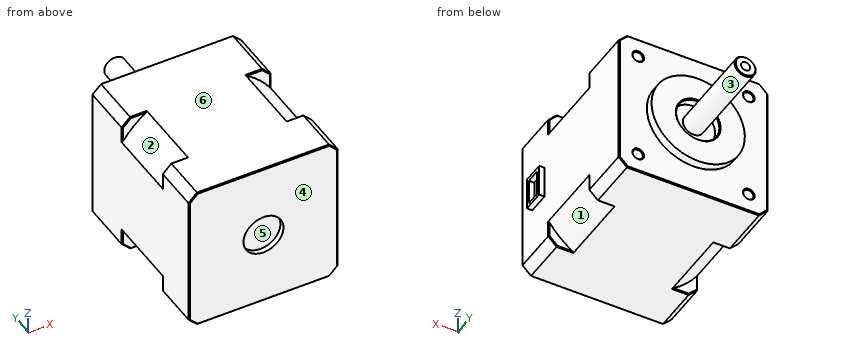
```python
from build123d import *

# Parameters (mm, degrees)
SKETCH1_W                = 35.052
SKETCH1_H                = 40.1574
BOSS_EXTRUDE1_DEPTH      = 35.052
CUT_EXTRUDE1_DEPTH       = 16.6878
CUT_EXTRUDE2_DEPTH       = 16.6878
CUT_EXTRUDE3_DEPTH       = 16.6878
CUT_EXTRUDE4_START       = -16.6878
CUT_EXTRUDE4_DEPTH       = 16.6878
SKETCH6_W                = 7.6708
SKETCH6_H                = 5.08
BOSS_EXTRUDE2_DEPTH      = 1.27
SKETCH7_W                = 5.999755797
SKETCH7_H                = 3.380210023
CUT_EXTRUDE5_DEPTH       = 1.27
SKETCH8_R                = 10.9728
BOSS_EXTRUDE3_DEPTH      = 1.9558
HOLE1_D                  = 10.16
HOLE1_DEPTH              = 1.9558
SKETCH11_W               = 2.5
SKETCH11_H               = 21.59
M8_CLEARANCE_HOLE1_D     = 9.398
M8_CLEARANCE_HOLE1_DEPTH = 1.27
M2_CLEARANCE_HOLE1_D     = 2.3876
M2_CLEARANCE_HOLE1_DEPTH = 7.62
HOLE2_D                  = 2.159089633
HOLE2_DEPTH              = 2.54
CHAMFER1_SIZE            = 2
CHAMFER2_SIZE            = 0.2


with BuildPart() as part:
    # Sketch1 → Boss-Extrude1 (new body)
    with BuildSketch(Plane(origin=(0, 0, 0), x_dir=(0, 0, -1), z_dir=(1, 0, 0))):
        with Locations((-17.526, 20.0787)):
            Rectangle(SKETCH1_W, SKETCH1_H)
    extrude(amount=-BOSS_EXTRUDE1_DEPTH)

    # Sketch2 → Cut-Extrude1 (cut)
    with BuildSketch(Plane(origin=(0, 27.7114, 0), x_dir=(1, 0, 0), z_dir=(0, 1, 0))):
        with BuildLine():
            Line((0, -5.923557746), (0, 0))
            Line((0, 0), (-5.923557746, 0))
            ThreePointArc((-5.923557746, 0), (-2.66367612, -2.66367612), (0, -5.923557746))
        make_face()
    extrude(amount=-CUT_EXTRUDE1_DEPTH, mode=Mode.SUBTRACT)

    # Sketch3 → Cut-Extrude2 (cut)
    with BuildSketch(Plane(origin=(0, 27.7114, 0), x_dir=(1, 0, 0), z_dir=(0, 1, 0))):
        with BuildLine():
            Line((-29.128442254, 0), (-35.052, 0))
            Line((-35.052, 0), (-35.052, -5.923557746))
            ThreePointArc((-35.052, -5.923557746), (-32.38832388, -2.66367612), (-29.128442254, 0))
        make_face()
    extrude(amount=-CUT_EXTRUDE2_DEPTH, mode=Mode.SUBTRACT)

    # Sketch4 → Cut-Extrude3 (cut)
    with BuildSketch(Plane(origin=(0, 27.7114, 0), x_dir=(1, 0, 0), z_dir=(0, 1, 0))):
        with BuildLine():
            Line((-35.052, -29.128442254), (-35.052, -35.052))
            Line((-35.052, -35.052), (-29.128442254, -35.052))
            ThreePointArc((-29.128442254, -35.052), (-32.38832388, -32.38832388), (-35.052, -29.128442254))
        make_face()
    extrude(amount=-CUT_EXTRUDE3_DEPTH, mode=Mode.SUBTRACT)

    # Sketch5 → Cut-Extrude4 (cut)
    with BuildSketch(Plane.XZ.offset(-11.0236).offset(CUT_EXTRUDE4_START)):
        with BuildLine():
            Line((0, 29.128442254), (0, 35.052))
            Line((0, 35.052), (-5.923557746, 35.052))
            ThreePointArc((-5.923557746, 35.052), (-2.66367612, 32.38832388), (0, 29.128442254))
        make_face()
    extrude(amount=CUT_EXTRUDE4_DEPTH, mode=Mode.SUBTRACT)

    # Sketch6 → Boss-Extrude2 (add)
    with BuildSketch(Plane(origin=(0, 0, 0), x_dir=(0, 0, -1), z_dir=(1, 0, 0))):
        with Locations((-17.526, 6.804)):
            Rectangle(SKETCH6_W, SKETCH6_H)
    extrude(amount=BOSS_EXTRUDE2_DEPTH)

    # Sketch7 → Cut-Extrude5 (cut)
    with BuildSketch(Plane(origin=(1.27, 0, 0), x_dir=(0, 0, -1), z_dir=(1, 0, 0))):
        with Locations((-17.472522102, 6.764894989)):
            Rectangle(SKETCH7_W, SKETCH7_H)
    extrude(amount=-CUT_EXTRUDE5_DEPTH, mode=Mode.SUBTRACT)

    # Sketch8 → Boss-Extrude3 (add)
    with BuildSketch(Plane(origin=(0, 40.1574, 0), x_dir=(-1, 0, 0), z_dir=(0, 1, 0))):
        with Locations(Location((17.526, 17.526, 0), (0, 0, 90))):
            Circle(SKETCH8_R)
    extrude(amount=BOSS_EXTRUDE3_DEPTH)

    # Hole1
    with Locations(Plane(origin=(0, 42.1132, 0), x_dir=(1, 0, 0), z_dir=(0, 1, 0))):
        with Locations((-17.526, -17.526)):
            Hole(HOLE1_D / 2, depth=HOLE1_DEPTH)

    # Sketch11 → Revolve1 (revolve)
    with BuildSketch(Plane(origin=(0, 0, 17.526), x_dir=(-1, 0, 0), z_dir=(0, 0, -1)), mode=Mode.PRIVATE) as revolve1_sk:
        with Locations((16.276, 50.9524)):
            Rectangle(SKETCH11_W, SKETCH11_H)
    revolve(revolve1_sk.sketch.rotate(Axis((-17.526, 40.1574, 17.526), (0, 1, 0)), 270), axis=Axis((-17.526, 40.1574, 17.526), (0, 1, 0)))

    # M8 Clearance Hole1
    with Locations(Plane(origin=(0, 0, 0), x_dir=(-1, 0, 0), z_dir=(0, -1, 0))):
        with Locations((17.526, -17.526)):
            Hole(M8_CLEARANCE_HOLE1_D / 2, depth=M8_CLEARANCE_HOLE1_DEPTH)

    # M2 Clearance Hole1
    with Locations(Plane(origin=(0, 40.1574, 0), x_dir=(1, 0, 0), z_dir=(0, 1, 0))):
        with Locations((-4.5308, -30.5212), (-30.5308, -4.5212), (-30.5308, -30.5212), (-4.5308, -4.5212)):
            Hole(M2_CLEARANCE_HOLE1_D / 2, depth=M2_CLEARANCE_HOLE1_DEPTH)

    # Hole2
    with Locations(Plane(origin=(0, 61.7474, 0), x_dir=(1, 0, 0), z_dir=(0, 1, 0))):
        with Locations((-17.526, -17.526)):
            Hole(HOLE2_D / 2, depth=HOLE2_DEPTH)

    # Chamfer1
    chamfer1_edges = [part.edges().sort_by_distance(p)[0] for p in [
        (-35.052, 5.5118, 0),
        (0, 33.9344, 0),
        (-35.052, 33.9344, 0),
        (-35.052, 5.5118, 35.052),
        (-35.052, 33.9344, 35.052),
        (0, 5.5118, 35.052),
        (0, 5.5118, 0),
        (0, 33.9344, 35.052),
    ]]
    chamfer(chamfer1_edges, length=CHAMFER1_SIZE)

    # Chamfer2
    chamfer2_edges = [part.edges().sort_by_distance(p)[0] for p in [
        (-3.337, 40.1574, 4.5212),
        (-29.337, 40.1574, 30.5212),
        (-29.337, 40.1574, 4.5212),
        (-3.337, 40.1574, 30.5212),
        (-3.961778873, 27.7114, 35.052),
        (-17.526, 40.1574, 35.052),
        (-31.090221127, 27.7114, 35.052),
        (-31.090221127, 11.0236, 35.052),
        (-17.526, 0, 35.052),
        (-3.961778873, 11.0236, 35.052),
        (-34.052, 27.7114, 34.052),
        (-35.052, 40.1574, 17.526),
        (-35.052, 27.7114, 3.961778873),
        (-35.052, 11.0236, 3.961778873),
        (-35.052, 0, 17.526),
        (0, 40.1574, 17.526),
        (-17.526, 40.1574, 0),
        (-1, 40.1574, 34.052),
        (-34.052, 40.1574, 1),
        (-1, 40.1574, 1),
        (-34.052, 40.1574, 34.052),
        (0, 0, 17.526),
        (-17.526, 0, 0),
        (-34.052, 0, 34.052),
        (-1, 0, 1),
        (-34.052, 0, 1),
        (-1, 0, 34.052),
        (-1, 11.0236, 34.052),
        (-3.961778873, 27.7114, 0),
        (-3.961778873, 11.0236, 0),
        (-34.052, 11.0236, 1),
        (-1, 27.7114, 1),
        (-1, 11.0236, 1),
        (-34.052, 27.7114, 1),
        (-1, 27.7114, 34.052),
        (-34.052, 11.0236, 34.052),
        (0, 11.0236, 3.961778873),
        (0, 27.7114, 3.961778873),
        (-31.090221127, 11.0236, 0),
        (-31.090221127, 27.7114, 0),
        (-35.052, 11.0236, 31.090221127),
        (-35.052, 27.7114, 31.090221127),
        (0, 27.7114, 31.090221127),
        (0, 11.0236, 31.090221127),
        (-12.446, 42.1132, 17.526),
        (-17.526, 61.7474, 15.026),
    ]]
    chamfer(chamfer2_edges, length=CHAMFER2_SIZE)


solid = part.part
```
Verification items for the finished model (mm, model axes). Face numbers are marked on the shaded views. A direction names the side the tool comes from. Give positions to 0.01 mm unless a question says otherwise; leave off trailing zeros. Order: outer loops, then holes, each group sorted by start corner. A loop starts at its lowest first (then second) coordinate and runs counter-clockwise, first axis right, second up. Notation, with made-up numbers: (32, 59) -> (70, 59) arc R7 ccw to (70, 68) -> close; hole circle Ø7 at (64, 26.5). An arc over 180 degrees is marked (long way). Use a Markdown table: item, result.
1) Section check D-D, the plane x = -24.5. Record the boundary of the cut face in (y, z), then the cut area to 3 significant figures.
Results:
| item | result |
|---|---|
| outline | (0, 0.2) -> (0.2, 0) -> (39.96, 0) -> (40.16, 0.2) -> (40.16, 9.05) -> (42.11, 9.05) -> (42.11, 26) -> (40.16, 26) -> (40.16, 34.85) -> (39.96, 35.05) -> (0.2, 35.05) -> (0, 34.85) -> close |
| area | 1,440 mm² |
2) Tool access check on the marked faces 1, 2 and 3. Record the directions out of +Z, -Z, +X, -X, +Y, -Y that give a thin tool (end or side, any length) a straight path to the whole face; none if there is none.
Results:
| item | result |
|---|---|
| face 1 | -Z, +X |
| face 2 | +Z, -X |
| face 3 | +Y |
3) Section check A-A, the plane y = 22. Record the boundary of the cut face in (x, z).
Results:
| item | result |
|---|---|
| outline | (-35.05, 5.92) arc R21.02 ccw to (-29.13, 0) -> (-5.92, 0) arc R21.02 ccw to (0, 5.92) -> (0, 29.13) arc R21.02 ccw to (-5.92, 35.05) -> (-29.13, 35.05) arc R21.02 ccw to (-35.05, 29.13) -> close |
4) Section check C-C, the plane x = -10. Record the boundary of the cut face in (y, z), then the cut area to 3 significant figures.
Results:
| item | result |
|---|---|
| outline | (0, 0.2) -> (0.2, 0) -> (39.96, 0) -> (40.16, 0.2) -> (40.16, 9.54) -> (42.11, 9.54) -> (42.11, 25.51) -> (40.16, 25.51) -> (40.16, 34.85) -> (39.96, 35.05) -> (0.2, 35.05) -> (0, 34.85) -> close |
| area | 1,440 mm² |
5) Material ranges on probe 1 along Y at (x, z) = (-4, 11); probe 2 along X at (y, z) = (27, 24); probe 3 along Y at (x, z) = (-24, 19), recorded low to high.
Results:
| item | result |
|---|---|
| probe 1 | 0 to 40.16 |
| probe 2 | -35.05 to 0 |
| probe 3 | 0 to 42.11 |
6) Depth check by flat-ended pin: pin 1 Ø1.2 at (x, z) = (-4, 4) entering from +Y; pin 2 Ø1.2 at (x, z) = (-5, 31) entering from +Y; pin 3 Ø0.7 at (x, z) = (-30.5, 5) entering from +Y; pin 4 Ø12 at (x, y) = (-6, 54.5) entering from -Z. Enter the tip coordinate at first touch or a pass-through.
Results:
| item | result |
|---|---|
| pin 1 | y = 40.11 |
| pin 2 | y = 40.03 |
| pin 3 | y = 32.54 |
| pin 4 | through |
7) Section check B-B, the plane y = 33.5. Record the boundary of the cut face in (x, z), then the cut area to 3 significant figures.
Results:
| item | result |
|---|---|
| outline | (-35.05, 2) -> (-33.05, 0) -> (-2, 0) -> (0, 2) -> (0, 33.05) -> (-2, 35.05) -> (-33.05, 35.05) -> (-35.05, 33.05) -> close; hole circle Ø2.39 at (-30.53, 4.52); hole circle Ø2.39 at (-30.53, 30.52); hole circle Ø2.39 at (-4.53, 4.52); hole circle Ø2.39 at (-4.53, 30.52) |
| area | 1,200 mm² |
8) Mould release check, pull along Z, two halves, no side actions. Record for the marked faces 4, 5 and 6: pulls with the +Z half, pulls with the -Z half, needs draft (parallel to the pull), parting line crosses it, or undercut.
Results:
| item | result |
|---|---|
| face 4 | needs draft |
| face 5 | undercut |
| face 6 | pulls with the +Z half |
